```python
from build123d import *

# Parameters (mm, degrees)
BOSS_EXTRUDE1_DEPTH = 9
FILLET1_R           = 2
CUT_EXTRUDE1_DEPTH  = 7
SKETCH3_R           = 1.1
CUT_EXTRUDE2_DEPTH  = 44.38862164
SKETCH4_R           = 1.5
BOSS_EXTRUDE2_DEPTH = 6
SKETCH5_R           = 1.1
CUT_EXTRUDE3_DEPTH  = 5
SKETCH7_R           = 1.21715418
BOSS_EXTRUDE3_DEPTH = 3
SKETCH8_W           = 16
SKETCH8_H           = 21
CUT_EXTRUDE4_DEPTH  = 3
SKETCH9_R           = 2
CUT_EXTRUDE5_DEPTH  = 54.392249766
SKETCH10_R          = 2.5
BOSS_EXTRUDE4_DEPTH = 2
SKETCH11_R          = 2
CUT_EXTRUDE6_DEPTH  = 43.738419489
SKETCH14_R          = 1.1
BOSS_EXTRUDE5_DEPTH = 3.5
SKETCH15_W          = 19
SKETCH15_H          = 15
CUT_EXTRUDE7_DEPTH  = 3.5
SKETCH16_W          = 1.21715418
SKETCH16_H          = 16.846199199
CUT_EXTRUDE8_DEPTH  = 3.5
SKETCH17_W          = 7.5
SKETCH17_H          = 3
CUT_EXTRUDE9_DEPTH  = 2.4


with BuildPart() as part:
    # Sketch1 → Boss-Extrude1 (new body)
    with BuildSketch(Plane(origin=(0, 0, 0), x_dir=(1, 0, 0), z_dir=(0, 1, 0))):
        with BuildLine():
            Line((-31.823529412, 18.890756303), (8.176470588, 18.890756303))
            ThreePointArc((8.176470588, 18.890756303), (11.712004494, 17.426290208), (13.176470588, 13.890756303))
            Line((13.176470588, 13.890756303), (13.176470588, -16.109243697))
            ThreePointArc((13.176470588, -16.109243697), (11.712004494, -19.644777603), (8.176470588, -21.109243697))
            Line((8.176470588, -21.109243697), (-31.823529412, -21.109243697))
            ThreePointArc((-31.823529412, -21.109243697), (-35.359063318, -19.644777603), (-36.823529412, -16.109243697))
            Line((-36.823529412, -16.109243697), (-36.823529412, 13.890756303))
            ThreePointArc((-36.823529412, 13.890756303), (-35.359063318, 17.426290208), (-31.823529412, 18.890756303))
        make_face()
    extrude(amount=BOSS_EXTRUDE1_DEPTH)

    # Fillet1
    fillet1_edges = [part.edges().sort_by_distance(p)[0] for p in [
        (11.712004494, 9, -17.426290208),
        (-11.823529412, 9, -18.890756303),
        (-35.359063318, 9, -17.426290208),
        (-36.823529412, 9, 1.109243697),
        (-35.359063318, 9, 19.644777603),
        (-11.823529412, 9, 21.109243697),
        (11.712004494, 9, 19.644777603),
        (13.176470588, 9, 1.109243697),
    ]]
    fillet(fillet1_edges, radius=FILLET1_R)

    # Sketch2 → Cut-Extrude1 (cut)
    with BuildSketch(Plane.XZ):
        with BuildLine():
            Line((-29.423529412, 18.709243697), (5.776470588, 18.709243697))
            ThreePointArc((5.776470588, 18.709243697), (9.312004494, 17.244777603), (10.776470588, 13.709243697))
            Line((10.776470588, 13.709243697), (10.776470588, -11.490756303))
            ThreePointArc((10.776470588, -11.490756303), (9.312004494, -15.026290208), (5.776470588, -16.490756303))
            Line((5.776470588, -16.490756303), (-29.423529412, -16.490756303))
            ThreePointArc((-29.423529412, -16.490756303), (-32.959063318, -15.026290208), (-34.423529412, -11.490756303))
            Line((-34.423529412, -11.490756303), (-34.423529412, 13.709243697))
            ThreePointArc((-34.423529412, 13.709243697), (-32.959063318, 17.244777603), (-29.423529412, 18.709243697))
        make_face()
    extrude(amount=-CUT_EXTRUDE1_DEPTH, mode=Mode.SUBTRACT)

    # Sketch3 → Cut-Extrude2 (cut, through all)
    with BuildSketch(Plane.XZ):
        with Locations(Location((10.376470588, 18.309243697, 0), (0, 0, 270))):
            Circle(SKETCH3_R)
        with Locations(Location((-34.023484676, 18.246215417, 0), (0, 0, 270))):
            Circle(SKETCH3_R)
        with Locations(Location((-34.023484676, -16.153784583, 0), (0, 0, 270))):
            Circle(SKETCH3_R)
        with Locations(Location((10.376470588, -16.090756303, 0), (0, 0, 270))):
            Circle(SKETCH3_R)
    extrude(amount=-CUT_EXTRUDE2_DEPTH, mode=Mode.SUBTRACT)

    # Sketch4 → Boss-Extrude2 (add)
    with BuildSketch(Plane.XZ.offset(-7)):
        with Locations(Location((6.201470588, 15.859243697, 0), (0, 0, 270))):
            Circle(SKETCH4_R)
        with Locations(Location((-30.298529412, 15.859243697, 0), (0, 0, 270))):
            Circle(SKETCH4_R)
        with Locations(Location((-30.298529412, -13.640756303, 0), (0, 0, 270))):
            Circle(SKETCH4_R)
        with Locations(Location((6.201470588, -13.640756303, 0), (0, 0, 270))):
            Circle(SKETCH4_R)
    extrude(amount=BOSS_EXTRUDE2_DEPTH)

    # Sketch5 → Cut-Extrude3 (cut)
    with BuildSketch(Plane.XZ.offset(-1)):
        with Locations(Location((6.201470588, 15.859243697, 0), (0, 0, 270))):
            Circle(SKETCH5_R)
        with Locations(Location((-30.298529412, 15.859243697, 0), (0, 0, 270))):
            Circle(SKETCH5_R)
        with Locations(Location((-30.298529412, -13.640756303, 0), (0, 0, 270))):
            Circle(SKETCH5_R)
        with Locations(Location((6.201470588, -13.640756303, 0), (0, 0, 270))):
            Circle(SKETCH5_R)
    extrude(amount=-CUT_EXTRUDE3_DEPTH, mode=Mode.SUBTRACT)

    # Sketch7 → Boss-Extrude3 (add)
    with BuildSketch(Plane(origin=(0, 7, 0), x_dir=(-1, 0, 0), z_dir=(0, -1, 0))):
        with Locations(Location((-4.201470588, -10.859243697, 0), (0, 0, 90))):
            Circle(SKETCH7_R)
        with Locations(Location((11.798529412, -10.859243697, 0), (0, 0, 90))):
            Circle(SKETCH7_R)
        with Locations(Location((11.798529412, 10.140756303, 0), (0, 0, 90))):
            Circle(SKETCH7_R)
        with Locations(Location((-4.201470588, 10.140756303, 0), (0, 0, 90))):
            Circle(SKETCH7_R)
    extrude(amount=BOSS_EXTRUDE3_DEPTH)

    # Sketch8 → Cut-Extrude4 (cut)
    with BuildSketch(Plane.XZ.offset(-4)):
        with Locations((-3.798529412, 0.359243697)):
            Rectangle(SKETCH8_W, SKETCH8_H)
    extrude(amount=-CUT_EXTRUDE4_DEPTH, mode=Mode.SUBTRACT)

    # Sketch9 → Cut-Extrude5 (cut, through all)
    with BuildSketch(Plane.XY.offset(-16.490756303)):
        with Locations((-24.423529412, 4)):
            Circle(SKETCH9_R)
    extrude(amount=-CUT_EXTRUDE5_DEPTH, mode=Mode.SUBTRACT)

    # Sketch10 → Boss-Extrude4 (add)
    with BuildSketch(Plane.XZ.offset(-7)):
        with Locations(Location((-4.423529412, 15.709243697, 0), (0, 0, 270))):
            Circle(SKETCH10_R)
    extrude(amount=BOSS_EXTRUDE4_DEPTH)

    # Sketch11 → Cut-Extrude6 (cut, through all)
    with BuildSketch(Plane.XZ.offset(-5)):
        with Locations(Location((-4.423529412, 15.709243697, 0), (0, 0, 270))):
            Circle(SKETCH11_R)
    extrude(amount=-CUT_EXTRUDE6_DEPTH, mode=Mode.SUBTRACT)

    # Sketch14 → Boss-Extrude5 (add)
    with BuildSketch(Plane(origin=(0, 7, 0), x_dir=(-1, 0, 0), z_dir=(0, -1, 0))):
        with Locations(Location((31.798529412, -10.859243697, 0), (0, 0, 90))):
            Circle(SKETCH14_R)
        with Locations(Location((31.798529412, 4.140756303, 0), (0, 0, 90))):
            Circle(SKETCH14_R)
        with Locations(Location((12.498529412, 4.140756303, 0), (0, 0, 90))):
            Circle(SKETCH14_R)
    extrude(amount=BOSS_EXTRUDE5_DEPTH)

    # Sketch15 → Cut-Extrude7 (cut)
    with BuildSketch(Plane.XZ.offset(-3.5)):
        with Locations((-22.298529412, 3.359243697)):
            Rectangle(SKETCH15_W, SKETCH15_H)
    extrude(amount=-CUT_EXTRUDE7_DEPTH, mode=Mode.SUBTRACT)

    # Sketch16 → Cut-Extrude8 (cut)
    with BuildSketch(Plane.XZ.offset(-3.5)):
        with Locations((-11.189952322, 2.436144097)):
            Rectangle(SKETCH16_W, SKETCH16_H)
    extrude(amount=-CUT_EXTRUDE8_DEPTH, mode=Mode.SUBTRACT)

    # Sketch17 → Cut-Extrude9 (cut)
    with BuildSketch(Plane.XY.offset(21.109243697)):
        with Locations((-20.316797715, 3.5)):
            Rectangle(SKETCH17_W, SKETCH17_H)
    extrude(amount=-CUT_EXTRUDE9_DEPTH, mode=Mode.SUBTRACT)


solid = part.part
```
Build history of the part. All positions in model axes, mm. A direction names the side the tool comes from. Round coordinates to 2 decimals unless told otherwise and drop trailing zeros. Order: outer loops, then holes, each group sorted by start corner. A loop starts at its lowest first (then second) coordinate and runs counter-clockwise, first axis right, second up. Notation, with made-up numbers: (-35, 37) - (-29, 37) arc R12 ccw to (-29, 49) - close; hole circle Ø9 at (74.5, -31.75). An arc over 180 degrees is marked (long way). Use a Markdown table: item, result.
1) Saw through at B-B on y = 7.75. Write the cut outline in (x, z), and give its area (3 significant figures).
Recorded:
| item | result |
|---|---|
| outline | (-36.68, -13.89) arc R4.85 ccw to (-31.82, -18.74) - (8.18, -18.74) arc R4.85 ccw to (13.03, -13.89) - (13.03, 16.11) arc R4.85 ccw to (8.18, 20.96) - (-31.82, 20.96) arc R4.85 ccw to (-36.68, 16.11) - close; hole circle Ø2.2 at (-34.02, -16.15); hole circle Ø2.2 at (-34.02, 18.25); hole circle Ø4 at (-4.42, 15.71); hole circle Ø2.2 at (10.38, -16.09); hole circle Ø2.2 at (10.38, 18.31) |
| area | 1,930 mm² |
2) Pull direction Z, two halves, no side cores. Call faces 4 (the face through (-12.1, 8.4, 20.54)), 5 (the face through (-36.25, 8.4, 0.9)), 6 (the face through (4.201, 5.5, -9.5)): pulls with the +Z half, pulls with the -Z half, needs draft (parallel to the pull), parting line crosses it, or undercut.
Recorded:
| item | result |
|---|---|
| face 4 | pulls with the +Z half |
| face 5 | needs draft |
| face 6 | undercut |
3) Wall check: L1, parallel to Z at x = -6.5, y = 3.5; L2, parallel to X at y = 3.25, z = -4; L3, parallel to X at y = 6, z = -9.5. Give the ranges that are in metal, low to high.
Recorded:
| item | result |
|---|---|
| L1 | z = -18.89 to -16.49, 18.71 to 21.11 |
| L2 | x = -36.82 to -34.42, 10.78 to 13.18 |
| L3 | x = -36.82 to -34.42, -12.83 to -11.8, 4.2 to 5.24, 10.78 to 13.18 |
4) Tool access for faces 1 (the face through (-12, 9, 1)), 2 (the face through (-12, 4, -10)), 3 (the face through (-16.567, 3, 20)): list every direction of +Z, -Z, +X, -X, +Y, -Y with a clear straight run to the whole face (end or side of a thin tool).
Recorded:
| item | result |
|---|---|
| face 1 | +Z, -Z, +X, -X, +Y |
| face 2 | -Y |
| face 3 | +Z |
5) Saw through at C-C on z = 1. Write the cut outline in (x, y).
Recorded:
| item | result |
|---|---|
| outline | (-36.82, 0) - (-34.42, 0) - (-34.42, 7) - (10.78, 7) - (10.78, 0) - (13.18, 0) - (13.18, 7) arc R2 ccw to (11.18, 9) - (-34.82, 9) arc R2 ccw to (-36.82, 7) - close |
6) Flat gauge pins, fed straight in: pin 1 Ø0.9 at (x, z) = (-13, -4) entering from -Y; pin 2 Ø1.5 at (x, z) = (-4.5, 9.5) entering from -Y; pin 3 Ø2.5 at (x, z) = (4, -10.5) entering from -Y; pin 4 Ø10 at (x, z) = (6, -1) entering from -Y. Where does each tip first touch, or does it go through?
Recorded:
| item | result |
|---|---|
| pin 1 | stops at y = 3.5 |
| pin 2 | stops at y = 7 |
| pin 3 | stops at y = 4 |
| pin 4 | stops at y = 0 |
7) Saw through at A-A on x = -18. Write the cut outline in (y, z), and give its area (3 significant figures).
Recorded:
| item | result |
|---|---|
| outline | (0, -18.89) - (7, -18.89) arc R2 ccw to (9, -16.89) - (9, 19.11) arc R2 ccw to (7, 21.11) - (5, 21.11) - (5, 18.71) - (7, 18.71) - (7, -16.49) - (0, -16.49) - close; (0, 18.71) - (2, 18.71) - (2, 21.11) - (0, 21.11) - close |
| area | 105 mm² |
8) Saw through at D-D on x = 2. Write the cut outline in (y, z), and give its area (3 significant figures).
Recorded:
| item | result |
|---|---|
| outline | (0, -18.89) - (7, -18.89) arc R2 ccw to (9, -16.89) - (9, 19.11) arc R2 ccw to (7, 21.11) - (0, 21.11) - (0, 18.71) - (7, 18.71) - (7, -16.49) - (0, -16.49) - close |
| area | 112 mm² |
